```python
from build123d import *

# Parameters (mm, degrees)
SKETCH2_W               = 80
SKETCH2_H               = 47.65
BOSS_EXTRUDE1_DEPTH     = 3.175
SKETCH3_W               = 15
SKETCH3_H               = 3.5
BOSS_EXTRUDE2_DEPTH     = 3.175
SKETCH4_W               = 3.5
SKETCH4_H               = 15
BOSS_EXTRUDE3_DEPTH     = 3.175
MIRROR2_COPY_1_SKETCH_W = 3.5
MIRROR2_COPY_1_SKETCH_H = 15
MIRROR2_COPY_1_DEPTH    = 3.175
MIRROR2_COPY_2_SKETCH_W = 3.5
MIRROR2_COPY_2_SKETCH_H = 15
MIRROR2_COPY_2_DEPTH    = 3.175
CUT_EXTRUDE1_DEPTH      = 10
MIRROR4_COPY_1_DEPTH    = 10
SKETCH6_W               = 13
SKETCH6_H               = 22
CUT_EXTRUDE2_DEPTH      = 52.468303353
FILLET1_R               = 1
FILLET1_OF_MIRROR5_R    = 1


with BuildPart() as part:
    # Sketch2 → Boss-Extrude1 (new body)
    with BuildSketch(Plane(origin=(0, 0, 0), x_dir=(1, 0, 0), z_dir=(0, 1, 0))):
        Rectangle(SKETCH2_W, SKETCH2_H)
    extrude(amount=BOSS_EXTRUDE1_DEPTH)

    # Sketch3 → Boss-Extrude2 (add)
    with BuildSketch(Plane(origin=(0, 3.175, 0), x_dir=(1, 0, 0), z_dir=(0, 1, 0))):
        with Locations((0, 25.575)):
            Rectangle(SKETCH3_W, SKETCH3_H)
    boss_extrude2 = extrude(amount=-BOSS_EXTRUDE2_DEPTH)

    # Sketch4 → Boss-Extrude3 (add)
    with BuildSketch(Plane(origin=(0, 3.175, 0), x_dir=(1, 0, 0), z_dir=(0, 1, 0))):
        with Locations((-41.75, 0)):
            Rectangle(SKETCH4_W, SKETCH4_H)
    boss_extrude3 = extrude(amount=-BOSS_EXTRUDE3_DEPTH)

    # Mirror1: Boss-Extrude3 across plane
    add(boss_extrude3.mirror(Plane(origin=(0, 0, 0), x_dir=(0, 0, 1), z_dir=(1, 0, 0))))

    # Mirror2: Boss-Extrude2 across plane
    add(boss_extrude2.mirror(Plane.XY))

    # Mirror2 copy 1 sketch → Mirror2 copy 1 (add)
    with BuildSketch(Plane(origin=(0, 3.175, 0), x_dir=(-1, 0, 0), z_dir=(0, 1, 0))):
        with Locations((-41.75, 0)):
            Rectangle(MIRROR2_COPY_1_SKETCH_W, MIRROR2_COPY_1_SKETCH_H)
    extrude(amount=-MIRROR2_COPY_1_DEPTH)

    # Mirror2 copy 2 sketch → Mirror2 copy 2 (add)
    with BuildSketch(Plane(origin=(0, 3.175, 0), x_dir=(1, 0, 0), z_dir=(0, 1, 0))):
        with Locations((-41.75, 0)):
            Rectangle(MIRROR2_COPY_2_SKETCH_W, MIRROR2_COPY_2_SKETCH_H)
    extrude(amount=-MIRROR2_COPY_2_DEPTH)

    # Sketch5 → Cut-Extrude1 (cut)
    with BuildSketch(Plane(origin=(0, 3.175, 0), x_dir=(1, 0, 0), z_dir=(0, 1, 0))):
        Polygon((-40, 13.55), (-36, 13.55), (-36, 14.55), (-32.5, 14.55), (-32.5, 10.45), (-36, 10.45), (-36, 11.45), (-40, 11.45), align=None)
    cut_extrude1 = extrude(amount=-CUT_EXTRUDE1_DEPTH, mode=Mode.SUBTRACT)

    # Mirror3: Cut-Extrude1 across plane
    add(cut_extrude1.mirror(Plane.XY), mode=Mode.SUBTRACT)

    # Mirror4: Cut-Extrude1 across plane
    add(cut_extrude1.mirror(Plane(origin=(0, 0, 0), x_dir=(0, 0, 1), z_dir=(1, 0, 0))), mode=Mode.SUBTRACT)

    # Mirror4 copy 1 sketch → Mirror4 copy 1 (cut)
    with BuildSketch(Plane(origin=(0, 3.175, 0), x_dir=(-1, 0, 0), z_dir=(0, 1, 0))):
        Polygon((-40, 13.55), (-36, 13.55), (-36, 14.55), (-32.5, 14.55), (-32.5, 10.45), (-36, 10.45), (-36, 11.45), (-40, 11.45), align=None)
    extrude(amount=-MIRROR4_COPY_1_DEPTH, mode=Mode.SUBTRACT)

    # Sketch6 → Cut-Extrude2 (cut, through all)
    with BuildSketch(Plane(origin=(0, 3.175, 0), x_dir=(1, 0, 0), z_dir=(0, 1, 0))):
        with Locations((11.5, 0)):
            Rectangle(SKETCH6_W, SKETCH6_H)
    cut_extrude2 = extrude(amount=-CUT_EXTRUDE2_DEPTH, mode=Mode.SUBTRACT)

    # Fillet1
    fillet1_edges = [part.edges().sort_by_distance(p)[0] for p in [
        (5, 1.5875, 11),
        (5, 1.5875, -11),
        (18, 1.5875, -11),
        (18, 1.5875, 11),
    ]]
    fillet(fillet1_edges, radius=FILLET1_R)

    # Mirror5: Cut-Extrude2 across plane
    add(cut_extrude2.mirror(Plane(origin=(0, 0, 0), x_dir=(0, 0, 1), z_dir=(1, 0, 0))), mode=Mode.SUBTRACT)

    # Fillet1 of Mirror5
    fillet1_of_mirror5_edges = [part.edges().sort_by_distance(p)[0] for p in [
        (-5, 1.5875, 11),
        (-5, 1.5875, -11),
        (-18, 1.5875, -11),
        (-18, 1.5875, 11),
    ]]
    fillet(fillet1_of_mirror5_edges, radius=FILLET1_OF_MIRROR5_R)


solid = part.part
```
Build history of the part. All positions in model axes, mm. A direction names the side the tool comes from. Round coordinates to 2 decimals unless told otherwise and drop trailing zeros. Write each loop counter-clockwise with the first axis right and the second up, starting at its lowest first coordinate (ties: lowest second). Pieces come first, ordered by that corner, then holes.
1) 3-axis set-ups, long thin cutter, end or side, ignore diameter. For faces 4 (the flat face through (40, 2, -9)), 5 (the flat face through (-40, 2, -19)), 6 (the flat face through (11, 2, -11)), 7 (the flat face through (38, 2, 13.55)): which of +Z, -Z, +X, -X, +Y, -Y reach the whole face in a straight line?
2) Pin check, flat tips, straight feed: pin 1 (1.6 mm diameter, centred on x = 27.5, y = 1, fed in from -Z) (3 decimals); pin 2 (1 mm diameter, centred on y = 1.5, z = -8.5, fed in from +X); pin 3 (0.8 mm diameter, centred on y = 1, z = -14, fed in from -X). Stop position of each tip, or through.
3) Mould opens along X. For faces 1 (the flat face through (38, 2, -11.45)), 2 (the flat face through (-40, 2, -9)), 3 (the flat face through (-34, 2, -14.55)) say: +X half, -X half, draft (parallel to the pull), parting line (faces both ways), or undercut.
4) Band-saw the part on D-D, the plane y = 1.1. Give the number of separate pieces and of enclosed holes in the cut face, and give its area (3 significant figures).
5) Band-saw the part on A-A, the plane x = -14. List the corners of the cut face in (y, z) (3 decimals).
6) Band-saw the part on C-C, the plane x = -37. List the corners of the cut face in (y, z) (3 decimals).
7) Drill centre lines: probe 1 along Z at (x, y) = (33, 2.1) (3 decimals); probe 2 along Z at (x, y) = (-37.5, 1.75) (3 decimals); probe 3 along X at (y, z) = (1.7, 14). Where is each one in solid material? Low to high.
8) Band-saw the part on B-B, the plane z = 6.5. List the corners of the cut face in (x, y) (3 decimals), and give its area (3 significant figures).
Ans:
1. face 4: -Z, +X, +Y, -Y
1. face 5: -Z, -X, +Y, -Y
1. face 6: +Y, -Y
1. face 7: +X, +Y, -Y
2. pin 1: stops at z = -23.825
2. pin 2: stops at x = 40
2. pin 3: stops at x = -40
3. face 1: draft
3. face 2: -X half
3. face 3: undercut
4. separate pieces: 1
4. enclosed holes: 2
4. area: 3,360 mm2
5. outline: (0, -23.825) - (3.175, -23.825) - (3.175, -11) - (0, -11) - close; (0, 11) - (3.175, 11) - (3.175, 23.825) - (0, 23.825) - close
6. outline: (0, -23.825) - (3.175, -23.825) - (3.175, -13.55) - (0, -13.55) - close; (0, -11.45) - (3.175, -11.45) - (3.175, 11.45) - (0, 11.45) - close; (0, 13.55) - (3.175, 13.55) - (3.175, 23.825) - (0, 23.825) - close
7. probe 1: z = -23.825 to -14.55, -10.45 to 10.45, 14.55 to 23.825
7. probe 2: z = -23.825 to -13.55, -11.45 to 11.45, 13.55 to 23.825
7. probe 3: x = -40 to -36, -32.5 to 32.5, 36 to 40
8. outline: (-43.5, 0) - (-18, 0) - (-18, 3.175) - (-43.5, 3.175) - close; (-5, 0) - (5, 0) - (5, 3.175) - (-5, 3.175) - close; (18, 0) - (43.5, 0) - (43.5, 3.175) - (18, 3.175) - close
8. area: 194 mm2
